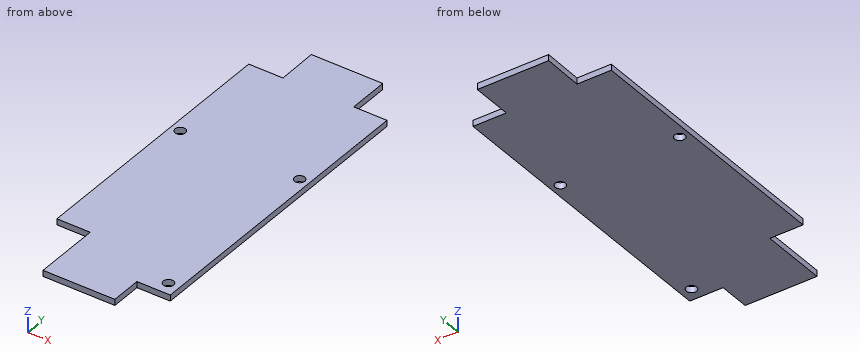
from build123d import *

# Parameters (mm, degrees)
BOSS_EXTRUDE1_DEPTH   = 1.5875
SKETCH2_W             = 8.73125
SKETCH2_H             = 9.2837
BOSS_EXTRUDE2_DEPTH   = 1.5875
F_2_CLEARANCE_HOLE1_D = 2.7051


with BuildPart() as part:
    # Sketch1 → Boss-Extrude1 (new body)
    with BuildSketch(Plane.XY):
        Polygon((-30.8483, -49.68875), (-30.8483, -98.31705), (-22.11705, -98.31705), (-22.11705, -115.77955), (-3.28295, -115.77955), (-3.28295, -98.31705), (5.4483, -98.31705), (5.4483, -49.68875), (5.4483, -27.41295), (-3.28295, -27.41295), (-3.28295, -16.66875), (-22.014883705, -16.66875), (-21.862168628, -27.33675), (-30.8483, -27.33675), align=None)
    extrude(amount=BOSS_EXTRUDE1_DEPTH)

    # Sketch2 → Boss-Extrude2 (add, through all)
    with BuildSketch(Plane.XY.offset(1.5875)):
        with Locations((1.082675, -102.9589)):
            Rectangle(SKETCH2_W, SKETCH2_H)
    extrude(amount=-BOSS_EXTRUDE2_DEPTH)

    # #2 Clearance Hole1 (through all)
    with Locations(Plane.XY.offset(1.5875)):
        with Locations((2.54, -104.14), (-28.336875, -56.1975), (2.936875, -56.1975)):
            Hole(F_2_CLEARANCE_HOLE1_D / 2)


solid = part.part
Verification items for the finished model (mm, model axes). Give positions to 0.01 mm unless a question says otherwise; leave off trailing zeros. Write each loop counter-clockwise with the first axis right and the second up, starting at its lowest first coordinate (ties: lowest second). Pieces come first, ordered by that corner, then holes.
(1) Cross-section at D-D (x = -25). Enter the section's corners in (y, z).
(2) Cross-section at C-C (x = 2.54). Enter the section's corners in (y, z), plus the area to 3 significant figures.
(3) Gauge pin test, flat ends, axial feed: pin 1 (0.5 mm diameter, centred on x = 0, z = 0.5, fed in from -Y); pin 2 (0.8 mm diameter, centred on x = 1.5, z = 0.5, fed in from +Y); pin 3 (0.5 mm diameter, centred on x = -27.5, z = 1, fed in from +Y). Record the tip position at first contact, or that the pin passes through.
(4) Material ranges on line 1 (X direction, y = -104.14, z = 0.7); line 2 (Y direction, x = 3, z = 0.2); line 3 (Y direction, x = 2, z = 1.4), recorded low to high.
(5) Cross-section at B-B (z = 0.35). Enter the section's corners in (x, y), plus the area to 3 significant figures.
(6) Cross-section at A-A (y = -104.14). Enter the section's corners in (x, z), plus the area to 3 significant figures.
Worked out:
1. outline: (-98.32, 0) - (-27.34, 0) - (-27.34, 1.59) - (-98.32, 1.59) - close
2. outline: (-107.6, 0) - (-105.49, 0) - (-105.49, 1.59) - (-107.6, 1.59) - close; (-102.79, 0) - (-57.49, 0) - (-57.49, 1.59) - (-102.79, 1.59) - close; (-54.9, 0) - (-27.41, 0) - (-27.41, 1.59) - (-54.9, 1.59) - close
2. area: 119 mm2
3. pin 1: stops at y = -107.6
3. pin 2: stops at y = -27.41
3. pin 3: stops at y = -27.34
4. line 1: x = -22.12 to 1.19, 3.89 to 5.45
4. line 2: y = -107.6 to -105.41, -102.87 to -57.55, -54.85 to -27.41
4. line 3: y = -107.6 to -105.38, -102.9 to -57.17, -55.22 to -27.41
5. outline: (-30.85, -98.32) - (-22.12, -98.32) - (-22.12, -115.78) - (-3.28, -115.78) - (-3.28, -107.6) - (5.45, -107.6) - (5.45, -27.41) - (-3.28, -27.41) - (-3.28, -16.67) - (-22.01, -16.67) - (-21.86, -27.34) - (-30.85, -27.34) - close; hole circle Ø2.71 at (-28.34, -56.2); hole circle Ø2.71 at (2.54, -104.14); hole circle Ø2.71 at (2.94, -56.2)
5. area: 3,170 mm2
6. outline: (-22.12, 0) - (1.19, 0) - (1.19, 1.59) - (-22.12, 1.59) - close; (3.89, 0) - (5.45, 0) - (5.45, 1.59) - (3.89, 1.59) - close
6. area: 39.5 mm2
